Input: part model. Units: mm. Frame: model coordinates. Coordinates: 2 decimals unless noted, no trailing zeros. Loops run counter-clockwise (first coordinate to the right, second up) from the corner with the lowest first, then second, coordinate; pieces in that order, holes last. Notation, with made-up numbers: (42.5, -20) - (78.5, -20) arc R7 ccw to (78.5, -11) - close; hole circle Ø2 at (-24.75, 63.5). An arc over 180 degrees is marked (long way). Use a Markdown table: item, result. Add a question column.
1. Section query C-C on x = 32. Return the cut outline in (y, z).
2. Section query D-D on x = -19. Return the cut outline in (y, z), then the cut area to 3 significant figures.
3. Ray query, L1, parallel to X at y = 1.2, z = -5; L2, parallel to X at y = 0.8, z = -1; L3, parallel to Z at x = -20, y = 0.85. Return the intervals inside material, ascending. Write a range as [from, to].
4. Section query B-B on z = -21. Return the cut outline in (x, y).
5. Section query A-A on y = 1.2. Return the cut outline in (x, z).
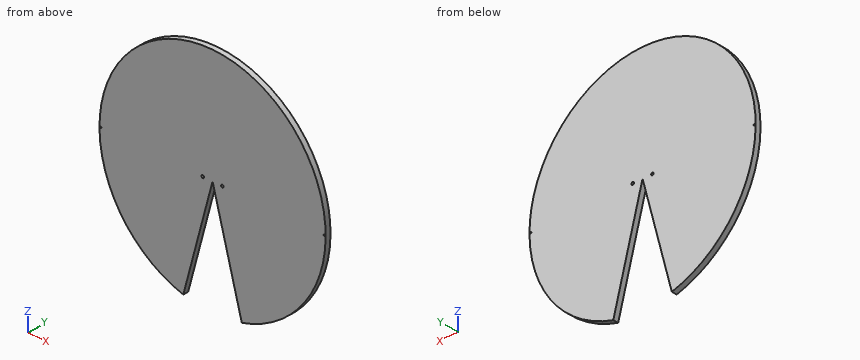
Autodesk Inventor part; units mm, degrees
ref_plane "Work Plane1" through (0, 1, 0) normal (0, 1, 0) x (-1, 0, 0)
ref_plane "YZ Plane" through (0, 0, 0) normal (1, 0, 0) x (0, 1, 0)
ref_plane "XY Plane" through (0, 0, 0) normal (0, 0, 1) x (1, 0, 0)
sketch "Sketch1" plane through (0, 0, 0) normal (0, 1, 0) x (-1, 0, 0)
  arc A0 (11.1292, -41.5348) -> (-11.1292, -41.5348) centre (0, 0) ccw
  line L0 (0, 0) -> (11.1292, -41.5348)
  line L1 (0, 0) -> (43, 0) construction
  line L2 (0, 0) -> (-11.1292, -41.5348)
  dimension "d0" = 86
  dimension "d1" = 75
extrude "Extrusion1" add sketch "Sketch1" along normal blind 2
ref_plane "Work Plane1" through (0, 1, 0) normal (0, 1, 0) x (-1, 0, 0)
sketch "Sketch2" plane through (0, 2, 0) normal (0, 1, 0) x (1, 0, 0)
  circle A0 centre (-42.5, 0) radius 0.25
  arc A1 (-11.1292, 41.5348) -> (11.1292, 41.5348) centre (0, 0) ccw
  dimension "d4" = 0.5
  dimension "d5" = 42.5
extrude "Extrusion2" cut sketch "Sketch2" against normal through all
mirror "Mirror1" about plane through (0, 0, 0) normal (1, 0, 0) of "Extrusion2"
sketch "Sketch4" plane through (0, 2, 0) normal (0, 1, 0) x (1, 0, 0)
  circle A0 centre (-3.75, 0) radius 0.5
  point P0 (0, 0)
  dimension "d12" = 1
  dimension "d13" = 3.75
extrude "Extrusion4" cut sketch "Sketch4" against normal through all
mirror "Mirror3" about plane through (0, 0, 0) normal (1, 0, 0) of "Extrusion4"
properties part number "seed_disp_lid" material "PMMA Plastic"
Resolved:
| question | item | result |
|---|---|---|
| 1 | outline | (0, -28.72) - (2, -28.72) - (2, 28.72) - (0, 28.72) - close |
| 2 | outline | (0, -38.57) - (2, -38.57) - (2, 38.57) - (0, 38.57) - close |
| 2 | area | 154 mm² |
| 3 | L1 | [-42.71, -1.34], [1.34, 42.71] |
| 3 | L2 | [-42.99, -0.27], [0.27, 42.99] |
| 3 | L3 | [-38.07, 38.07] |
| 4 | outline | (-37.52, 0) - (-5.63, 0) - (-5.63, 2) - (-37.52, 2) - close; (5.63, 0) - (37.52, 0) - (37.52, 2) - (5.63, 2) - close |
| 5 | outline | (-11.13, -41.53) - (0, 0) - (11.13, -41.53) arc R43 ccw (long way) to start; hole circle Ø0.5 at (-42.5, 0); hole circle Ø1 at (-3.75, 0); hole circle Ø1 at (3.75, 0); hole circle Ø0.5 at (42.5, 0) |
